Check sheet for the drawn part. Datum: minimum x, y, z corner. Units: mm. Give positions to 0.01 mm unless a question says otherwise; leave off trailing zeros. Order: outer loops, then holes, each group sorted by start corner. A loop starts at its lowest first (then second) coordinate and runs counter-clockwise, first axis right, second up.
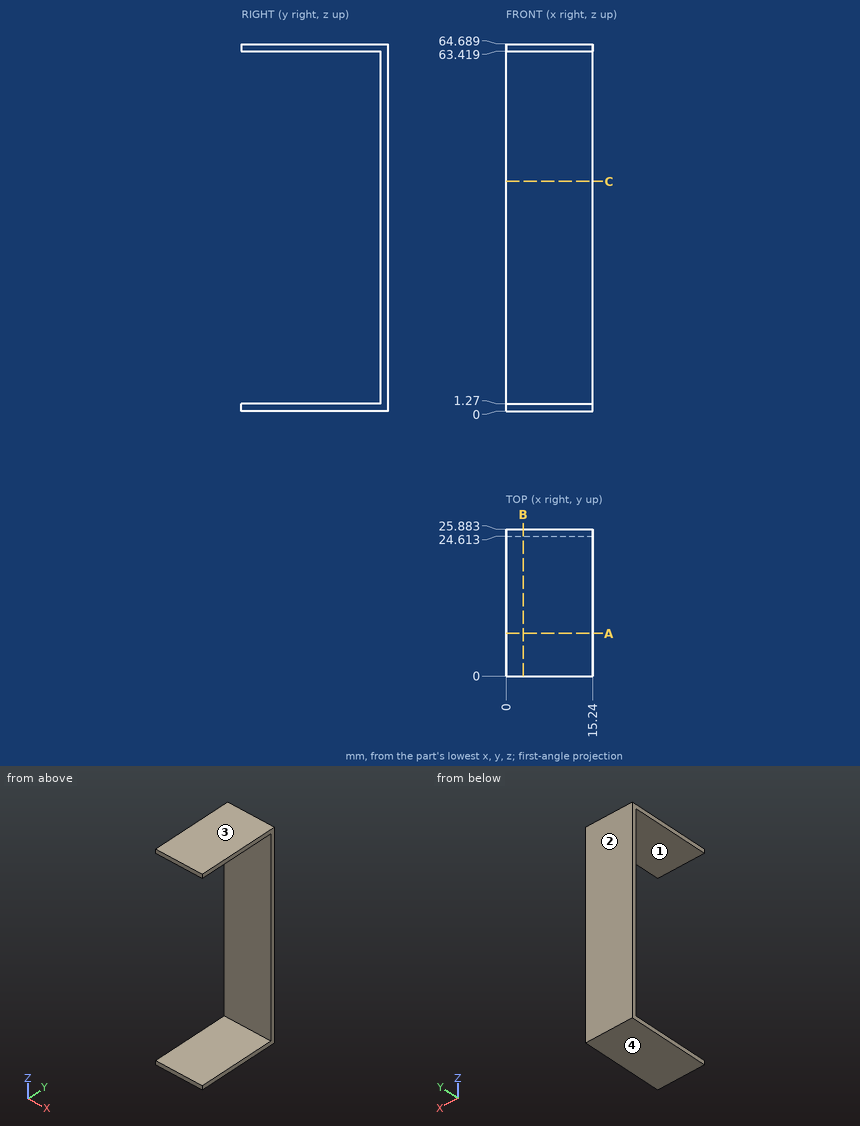
(1) Release check for a two-part mould opening along Z. For the marked faces 1, 2, 3 and 4 record: pulls with the +Z half, pulls with the -Z half, needs draft (parallel to the pull), parting line crosses it, or undercut.
Solved:
face 1: undercut
face 2: needs draft
face 3: pulls with the +Z half
face 4: pulls with the -Z half
(2) Section check C-C, the plane z = 40.5. Enter the section's corners in (x, y).
Solved:
outline: (0, 24.61) - (15.24, 24.61) - (15.24, 25.88) - (0, 25.88) - close
(3) Go/stop test with flat-tipped pins: pin 1 (6 mm diameter, centred on x = 11.5, z = 33, fed in from -Y); pin 2 (10 mm diameter, centred on y = 20.5, z = 15.5, fed in from +X). Record where each tip stops, or that it passes through.
Solved:
pin 1: stops at y = 24.61
pin 2: stops at x = 15.24
(4) Section check A-A, the plane y = 7.5. Enter the section's corners in (x, z).
Solved:
outline: (0, 0) - (15.24, 0) - (15.24, 1.27) - (0, 1.27) - close; (0, 63.42) - (15.24, 63.42) - (15.24, 64.69) - (0, 64.69) - close
(5) Scan lines: line 1 (Z direction, x = 14, y = 4); line 2 (Y direction, x = 5.5, z = 27.5). Record each from-to range of solid material in increasing order.
Solved:
line 1: z = 0 to 1.27, 63.42 to 64.69
line 2: y = 24.61 to 25.88
(6) Section check B-B, the plane x = 3. Enter the section's corners in (y, z).
Solved:
outline: (0, 0) - (25.88, 0) - (25.88, 64.69) - (0, 64.69) - (0, 63.42) - (24.61, 63.42) - (24.61, 1.27) - (0, 1.27) - close
